Design review of the part built by this model. Coordinates are the model's own, in mm. A direction names the side the tool comes from. Give positions to 0.01 mm unless a question says otherwise; leave off trailing zeros. Loops run counter-clockwise (first coordinate to the right, second up) from the corner with the lowest first, then second, coordinate; pieces in that order, holes last. Notation, with made-up numbers: M 42,72 L 46,72 A17 cw 46,95 Z; hole C 15.5,-4.5 d4. An arc over 180 degrees is marked long. Answer as CSV lines item,"result".
```python
from build123d import *

# Parameters (mm, degrees)
BOSS_EXTRUDE1_DEPTH = 1
SKETCH2_R           = 4
CUT_EXTRUDE1_DEPTH  = 58.046034043
FILLET1_R           = 5
FILLET2_R           = 2.5


with BuildPart() as part:
    # Sketch1 → Boss-Extrude1 (new, symmetric)
    with BuildSketch(Plane.XY):
        with BuildLine():
            Line((-38, 4), (-18.062391868, 4))
            ThreePointArc((-18.062391868, 4), (0, 18.5), (18.062391868, 4))
            Line((18.062391868, 4), (38, 4))
            Line((38, 4), (38, 19.032866311))
            ThreePointArc((38, 19.032866311), (0, 42.5), (-38, 19.032866311))
            Line((-38, 19.032866311), (-38, 4))
        make_face()
    extrude(amount=BOSS_EXTRUDE1_DEPTH, both=True)

    # Sketch2 → Cut-Extrude1 (cut, through all)
    with BuildSketch(Plane.XY.offset(1)):
        with Locations((-27.349588662, 13.5)):
            Circle(SKETCH2_R)
        with Locations((-19.442222095, 23.5)):
            Circle(SKETCH2_R)
        with Locations((19.442222095, 23.5)):
            Circle(SKETCH2_R)
        with Locations((27.349588662, 13.5)):
            Circle(SKETCH2_R)
    extrude(amount=-CUT_EXTRUDE1_DEPTH, mode=Mode.SUBTRACT)

    # Fillet1
    fillet1_edges = [part.edges().sort_by_distance(p)[0] for p in [
        (38, 4, 0),
        (-38, 4, 0),
    ]]
    fillet(fillet1_edges, radius=FILLET1_R)

    # Fillet2
    fillet2_edges = [part.edges().sort_by_distance(p)[0] for p in [
        (-38, 19.032866311, 0),
        (38, 19.032866311, 0),
        (18.062391868, 4, 0),
        (-18.062391868, 4, 0),
    ]]
    fillet(fillet2_edges, radius=FILLET2_R)


solid = part.part
```
1. We need section C-C, the plane y = 7. Write out the cut boundary in (x, z).
Answer block:
outline,"M -37.58,-1 L -17.12,-1 L -17.12,1 L -37.58,1 Z; M 17.12,-1 L 37.58,-1 L 37.58,1 L 17.12,1 Z"
2. We need section D-D, the plane y = 23.5. Write out the cut boundary in (x, z), plus the area to 3 significant figures.
Answer block:
outline,"M -35.41,-1 L -23.44,-1 L -23.44,1 L -35.41,1 Z; M -15.44,-1 L 15.44,-1 L 15.44,1 L -15.44,1 Z; M 23.44,-1 L 35.41,-1 L 35.41,1 L 23.44,1 Z"
area,"110 mm²"
3. We need section A-A, the plane z = 0.25. Write out the cut boundary in (x, y).
Answer block:
outline,"M -38,9 A5 ccw -33,4 L -19.97,4 A2.5 ccw -17.59,5.73 A18.5 cw 17.59,5.73 A2.5 ccw 19.97,4 L 33,4 A5 ccw 38,9 L 38,18.43 A2.5 ccw 37.72,19.58 A42.5 ccw -37.72,19.58 A2.5 ccw -38,18.43 Z; hole C -27.35,13.5 d8; hole C -19.44,23.5 d8; hole C 19.44,23.5 d8; hole C 27.35,13.5 d8"
4. To check wall thickness, follow L1, parallel to X at y = 13, z = 0.5; L2, parallel to X at y = 26.5, z = -0.8; L3, parallel to X at y = 24.5, z = -0.35. State the ranges of each line that lie inside material, in increasing order. Write a range as [from, to].
Answer block:
L1,"[-38, -31.32], [-23.38, -13.16], [13.16, 23.38], [31.32, 38]"
L2,"[-33.23, -22.09], [-16.8, 16.8], [22.09, 33.23]"
L3,"[-34.73, -23.32], [-15.57, 15.57], [23.32, 34.73]"
5. For faces 1 (the cylindrical face through (-18.518, 4.464, 0.014)), 2 (the flat face through (-1, 24, 1)), list the 3-axis set-ups (+Z, -Z, +X, -X, +Y, -Y) from which the entire face can be reached by the end or side of a thin tool; tool diameter is ignored.
Answer block:
face 1,"+Z, -Z, -Y"
face 2,"+Z, +X, -X, +Y, -Y"
6. The part is to be moulded in two halves that separate along Y. For faces 3 (the cylindrical face through (0.65, 42.495, 0.014)), 4 (the cylindrical face through (16.49, 26.2, 0.01)), 5 (the cylindrical face through (18.48, 4.49, 0.01)), say which applies: pulls with the +Y half, pulls with the -Y half, needs draft (parallel to the pull), parting line crosses it, or undercut.
Answer block:
face 3,"pulls with the +Y half"
face 4,"undercut"
face 5,"pulls with the -Y half"
7. We need section B-B, the plane y = 12.5. Write out the cut boundary in (x, z), plus the area to 3 significant figures.
Answer block:
outline,"M -38,-1 L -31.22,-1 L -31.22,1 L -38,1 Z; M -23.48,-1 L -13.64,-1 L -13.64,1 L -23.48,1 Z; M 13.64,-1 L 23.48,-1 L 23.48,1 L 13.64,1 Z; M 31.22,-1 L 38,-1 L 38,1 L 31.22,1 Z"
area,"66.5 mm²"
